```python
from build123d import *

# Parameters (mm, degrees)
SKETCH1_R               = 2
BOSS_EXTRUDE1_DEPTH     = 12
CUT_EXTRUDE1_REACH      = 63.528
CUT_EXTRUDE1_END_RADIUS = 5.25
SKETCH2_R               = 1.25
CUT_EXTRUDE2_REACH      = 45.868
CUT_EXTRUDE2_END_RADIUS = 25
CUT_EXTRUDE2_START      = -6
SKETCH3_R               = 3
CUT_EXTRUDE3_DEPTH      = 38.868128668
CUT_EXTRUDE3_DEPTH_BACK = 38.868128668
SKETCH3_4_R             = 1.5
CUT_EXTRUDE4_REACH      = 50.868
CUT_EXTRUDE4_END_RADIUS = 25
CUT_EXTRUDE4_START      = 11
FILLET1_R               = 2


with BuildPart() as part:
    # Sketch1 → Boss-Extrude1 (new body)
    with BuildSketch(Plane(origin=(0, 0, 0), x_dir=(1, 0, 0), z_dir=(0, 1, 0))):
        with BuildLine():
            ThreePointArc((-24.987593797, -0.7875), (25, 0), (-24.987593797, 0.7875))
            Line((-24.987593797, 0.7875), (-5.190601482, 0.7875))
            ThreePointArc((-5.190601482, 0.7875), (5.25, 0), (-5.190601482, -0.7875))
            Line((-5.190601482, -0.7875), (-24.987593797, -0.7875))
        make_face()
        with Locations(Location((0, 20, 0), (0, 0, 270))):
            Circle(SKETCH1_R, mode=Mode.SUBTRACT)
        with Locations(Location((20, 0, 0), (0, 0, 270))):
            Circle(SKETCH1_R, mode=Mode.SUBTRACT)
        with Locations(Location((0, -20, 0), (0, 0, 270))):
            Circle(SKETCH1_R, mode=Mode.SUBTRACT)
    extrude(amount=BOSS_EXTRUDE1_DEPTH)

    # Cut-Extrude1: up to this cylinder (the profile starts outside it)
    cut_extrude1_end = Plane(origin=(0, 4.5, 0), z_dir=(0, -1, 0)) * Cylinder(CUT_EXTRUDE1_END_RADIUS, 138.556, mode=Mode.PRIVATE)
    # Sketch2 → Cut-Extrude1 (cut, up to the surface)
    with BuildSketch(Plane(origin=(17.67766953, 0, 17.67766953), x_dir=(0, -1, 0), z_dir=(0.7071067811865464, 0, 0.7071067811865488)), mode=Mode.PRIVATE) as cut_extrude1_sk1:
        with Locations(Location((-4.5, 0, 0), (0, 0, 90))):
            Circle(SKETCH2_R)
    cut_extrude1_tool1 = extrude(cut_extrude1_sk1.sketch, amount=-CUT_EXTRUDE1_REACH, mode=Mode.PRIVATE) - cut_extrude1_end
    add(cut_extrude1_tool1.solids().sort_by_distance((17.67767, 4.5, 17.67767))[0], mode=Mode.SUBTRACT)

    # Cut-Extrude2: up to this cylinder (the profile starts inside it)
    cut_extrude2_end = Plane(origin=(0, 6, 0), z_dir=(0, -1, 0)) * Cylinder(CUT_EXTRUDE2_END_RADIUS, 142.736, mode=Mode.PRIVATE)
    # Sketch3 → Cut-Extrude2 (cut, up to the surface)
    with BuildSketch(Plane.XY.offset(-0.7875).offset(CUT_EXTRUDE2_START), mode=Mode.PRIVATE) as cut_extrude2_sk1:
        with Locations((-17.487593797, 6)):
            Circle(SKETCH3_R)
    cut_extrude2_tool1 = extrude(cut_extrude2_sk1.sketch, amount=-CUT_EXTRUDE2_REACH, mode=Mode.PRIVATE) & cut_extrude2_end
    add(cut_extrude2_tool1.solids().sort_by_distance((-17.487594, 6, -6.7875))[0], mode=Mode.SUBTRACT)

    # Sketch3<4> → Cut-Extrude3 (cut, two sides: drawn at the far end of the back side and taken through both)
    with BuildSketch(Plane.XY.offset(-0.7875).offset(-CUT_EXTRUDE3_DEPTH_BACK)):
        with Locations((-17.487593797, 6)):
            Circle(SKETCH3_4_R)
    extrude(amount=CUT_EXTRUDE3_DEPTH + CUT_EXTRUDE3_DEPTH_BACK, mode=Mode.SUBTRACT)

    # Cut-Extrude4: up to this cylinder (the profile starts inside it)
    cut_extrude4_end = Plane(origin=(0, 6, 0), z_dir=(0, -1, 0)) * Cylinder(CUT_EXTRUDE4_END_RADIUS, 152.736, mode=Mode.PRIVATE)
    # Sketch5 → Cut-Extrude4 (cut, up to the surface)
    with BuildSketch(Plane.XY.offset(-0.7875).offset(CUT_EXTRUDE4_START), mode=Mode.PRIVATE) as cut_extrude4_sk1:
        Polygon((-14.987593797, 7.443375673), (-17.487593797, 8.886751346), (-19.987593797, 7.443375673), (-19.987593797, 4.556624327), (-17.487593797, 3.113248654), (-14.987593797, 4.556624327), align=None)
    cut_extrude4_tool1 = extrude(cut_extrude4_sk1.sketch, amount=CUT_EXTRUDE4_REACH, mode=Mode.PRIVATE) & cut_extrude4_end
    add(cut_extrude4_tool1.solids().sort_by_distance((-17.487594, 6, 10.2125))[0], mode=Mode.SUBTRACT)

    # Fillet1
    fillet1_edges = [part.edges().sort_by_distance(p)[0] for p in [
        (25, 0, 0),
    ]]
    fillet(fillet1_edges, radius=FILLET1_R)


solid = part.part
```
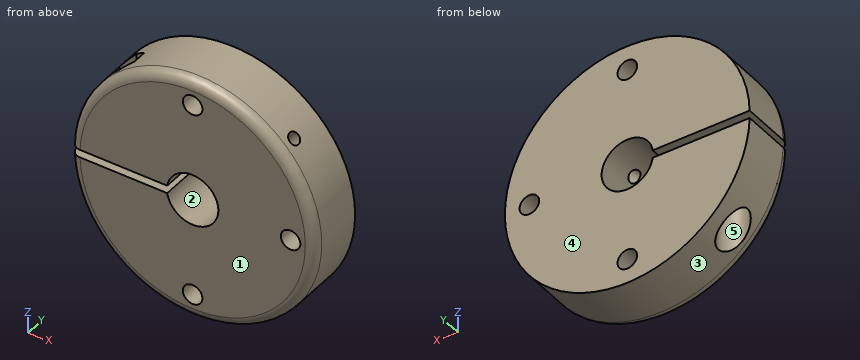
Work out the finished part from the listing and answer in its coordinate system (mm). Face numbers are marked on the shaded views. A direction names the side the tool comes from. Give positions to 0.01 mm unless a question says otherwise; leave off trailing zeros. Loops run counter-clockwise (first coordinate to the right, second up) from the corner with the lowest first, then second, coordinate; pieces in that order, holes last. Notation, with made-up numbers: (86, -30) - (136, -30) arc R25 ccw to (136, -5) - close; hole circle Ø1 at (65, -1). An arc over 180 degrees is marked (long way). One line per question, with ' | ' between items.
(1) Straight lines are drawn through the part: probe 1 along X at (y, z) = (6, -2.1); probe 2 along X at (y, z) = (6.75, -1.5); probe 3 along X at (y, z) = (6, -5.3). For each, find the intervals that lie inside material, in ascending order.
Recorded:
probe 1: x = -24.91 to -18.99, -15.99 to -4.81, 4.81 to 24.91 | probe 2: x = -24.95 to -18.79, -16.19 to -5.03, 5.03 to 18.68, 21.32 to 24.95 | probe 3: x = -24.43 to -18.99, -15.99 to 24.43
(2) The part is cut by section B-B (y = 11). Write down the section's boundary in (x, z), then the cut area to 3 significant figures.
Recorded:
outline: (-24.99, -0.79) arc R25 ccw (long way) to (-24.99, 0.79) - (-5.19, 0.79) arc R5.25 cw (long way) to (-5.19, -0.79) - close; hole circle Ø4 at (0, -20); hole circle Ø4 at (0, 20); hole circle Ø4 at (20, 0) | area: 1,810 mm²
(3) A tool of negligible diameter and unlimited length cuts with its end or side. For the marked faces 4 and 5, from which of +Z, -Z, +X, -X, +Y, -Y can it reach the whole face along a straight path? Write none if from no direction.
Recorded:
face 4: +Z, -Z, +X, -X, +Y | face 5: -Z
(4) Each of these flat-tipped pins is pushed along its axis until it touches: pin 1 Ø1.5 at (x, y) = (18.5, 2.5) entering from -Z; pin 2 Ø4 at (x, y) = (-17.49, 6) entering from +Z; pin 3 Ø2.5 at (y, z) = (6.5, 17) entering from -X. Where does it stop, or does it pass through?
Recorded:
pin 1: stops at z = -17.61 | pin 2: stops at z = 10.21 | pin 3: stops at x = -15.52
(5) The part is cut by section A-A (z = 0). Write down the section's boundary in (x, y), then the cut area to 3 significant figures.
Recorded:
outline: (5.25, 0) - (18, 0) - (18, 12) - (5.25, 12) - close; (22, 0) - (23, 0) arc R2 ccw to (25, 2) - (25, 12) - (22, 12) - close | area: 188 mm²
(6) The mould has two halves that part along X. Classify the marked faces 1, 2 and 3: +X half, -X half, draft (parallel to the pull), parting line (faces both ways), or undercut.
Recorded:
face 1: draft | face 2: undercut | face 3: parting line
(7) The part is cut by section C-C (x = 0). Count the separate pieces of the cut face and the enclosed holes in it, then the cut area to 3 significant figures.
Recorded:
separate pieces: 4 | enclosed holes: 0 | area: 376 mm²
